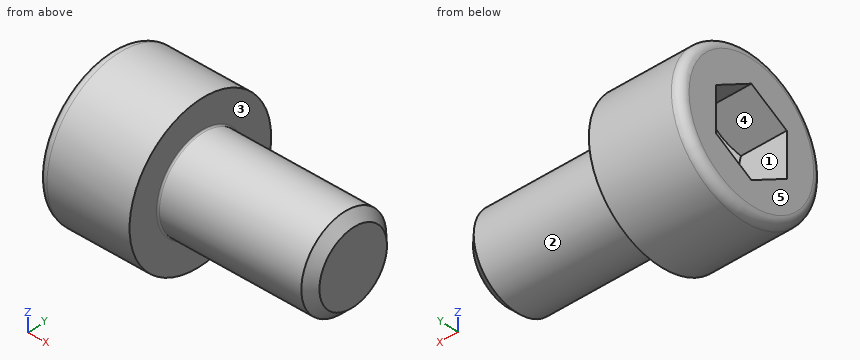
Autodesk Inventor part; units mm, degrees
ref_plane "Work Plane1" through (29, 0, 0) normal (0, -1, 0) x (1, 0, 0)
ref_plane "YZ Plane" through (0, 0, 0) normal (1, 0, 0) x (0, 1, 0)
ref_plane "XZ Plane" through (0, 0, 0) normal (0, 1, 0) x (-1, 0, 0)
sketch "Sketch1" plane through (0, 0, 0) normal (0, 0, 1) x (1, 0, 0)
  line L0 (-1.3333, 0) -> (10, 0)
  line L1 (10, 0) -> (10, 3)
  line L2 (10, 3) -> (2.5, 3)
  line L3 (2.5, 3) -> (1.8865, 3)
  line L4 (1.8865, 3) -> (0, 3)
  line L5 (0, 3) -> (0, 5)
  line L6 (0, 5) -> (-6, 5)
  line L7 (-6, 5) -> (-6, 2.8868)
  line L8 (-6, 2.8868) -> (-3, 2.8868)
  line L9 (-3, 2.8868) -> (-1.3333, 0)
  line L10 (-9.2, 0) -> (13.2, 0)
  line L11 (0, -1) -> (0, 6)
  line L12 (2.5, 3) -> (0, 3) construction
  dimension "d1" = 7.5
  dimension "d2" = 0.6136
  dimension "d3" = 6
  dimension "d4" = 3
  dimension "d5" = 60
  dimension "d6" = 6
  dimension "d7" = 6
  dimension "d8" = 5.7735
  dimension "d9" = 10
  dimension "d26" = 10
revolve "Body" add sketch "Sketch1" angle 360 about axis through (-1.3333, 0, 0) along (1, 0, 0)
sketch "Sketch2" plane through (-6, 0, 0) normal (-1, 0, 0) x (0, 0, 1)
  circle A0 centre (0, 0) radius 2.8868
  line L0 (0, -7) -> (0, 7)
  line L1 (-7, 0) -> (7, 0)
  line L2 (2.8868, 0) -> (1.4434, -2.5)
  line L3 (1.4434, -2.5) -> (-1.4434, -2.5)
  line L4 (-1.4434, -2.5) -> (-2.8868, 0)
  line L5 (-2.8868, 0) -> (-1.4434, 2.5)
  line L6 (-1.4434, 2.5) -> (1.4434, 2.5)
  line L7 (1.4434, 2.5) -> (2.8868, 0)
extrude "Slot" add sketch "Sketch2" against normal up to next contours L7 A0 | A0 L2 | L6 L0 A0 | A0 L0 L3 | L0 L6 A0 | A0 L3 L0 | L4 A0 | A0 L5
fillet "Fillet1" radius 0.6 1 edges at (-6, -5, 0)
thread "Thread"
chamfer "Chamfer1" distance 0.6135 distance2 0.6135 1 edges at (10, -3, 0) measured on face at (10, 0.705, 0.3049)
ref_plane "Work Plane1" through (29, 0, 0) normal (0, -1, 0) x (1, 0, 0)
fillet "Fillet2" radius 0.1 1 edges at (0, -3, 0)
equation "\"d1\" = GEL"
equation "\"d3\" = KOH"
equation "\"d4\" = INTI"
equation "\"d6\" = GD"
equation "\"d7\" = BDM"
equation "\"d8\" = 1.1547 * SW"
equation "\"d9\" = KOD"
equation "\"d26\" = NLG"
equation "\"d30\" = R"
equation "\"d17\" = RR"
equation "\"d13\" = GEL"
equation "\"d15\" = -0.5 * SPD + 0.5 * GD"
equation "\"d16\" = GUL"
equation "\"GD\" = NND"
equation "\"NLG\" = 10"
equation "\"GEL\" = 7.5"
equation "\"KOD\" = 10"
equation "\"KOH\" = NND"
equation "\"INTI\" = 3"
equation "\"GAL\" = 0.61345 * PTC"
equation "\"GUL\" = 0.61345 * PTC"
equation "\"BDM\" = NND"
equation "\"SW\" = 5"
equation "\"RR\" = 0.1 * NND"
equation "\"SPD\" = NND - 1.2269 * PTC"
equation "\"R\" = 0.1"
equation "\"PHH\" = 0.2"
equation "\"GD1\" = THREADDIA - 1.2269 * PTC"
equation "\"THREADDIA\" = 6"
equation "\"FAWI\" = 45deg"
equation "\"PTC\" = 1"
equation "\"KOH1\" = 5.4"
equation "\"NND\" = 6"
equation "\"TOA\" = 30deg"
equation "\"E0\" = 1.155 * SW"
properties part number "AS 1420 - 1973 - M6 x 10" material "Steel, Mild"
The listing builds one solid part. Answer for the finished solid, in the listing's coordinates (mm). Face numbers are marked on the shaded views. A direction names the side the tool comes from. Round coordinates to 2 decimals unless told otherwise and drop trailing zeros. Order: outer loops, then holes, each group sorted by start corner. A loop starts at its lowest first (then second) coordinate and runs counter-clockwise, first axis right, second up. Notation, with made-up numbers: M 53.25,34 L 66.25,34 A32 ccw 66.25,66 Z; hole C -20.75,-26.75 d5. An arc over 180 degrees is marked long. Answer in a Markdown table with one row per item. Add a question column.
1) Consider line 1 along X through (y, z) = (2.5, -2.25); line 2 along Y through (x, z) = (-2.5, 4); line 3 along Y through (x, z) = (-4.25, -0.5). Determine where each line is inside the solid, lowest interval first. Write a range as from..to.
2) The part is cut by section B-B on x = -1. Determine the outline of the cut face in (y, z).
3) Determine the mould class of the marked faces 1, 2 and 3 for opening direction Y: pulls with the +Y half, pulls with the -Y half, needs draft (parallel to the pull), parting line crosses it, or undercut.
4) Flat-ended cylindrical pins translate along their axes: pin 1 Ø1 at (y, z) = (1, 1.5) entering from -X; pin 2 Ø1.5 at (x, y) = (-2.5, 2.5) entering from -Z; pin 3 Ø1 at (x, z) = (4.5, 1) entering from -Y. Find the tip coordinate at first contact, or state that the pin passes through.
5) Which of the six approach directions +Z, -Z, +X, -X, +Y, -Y give full straight-line access (tool end or side, diameter ignored) to the marked faces 4 and 5?
6) The part is cut by section A-A on x = -3.5. Determine the outline of the cut face in (y, z).
Findings below:
| question | item | result |
|---|---|---|
| 1 | line 1 | x = -6..0 |
| 1 | line 2 | y = -3..3 |
| 1 | line 3 | y = -4.97..-2.5, 2.5..4.97 |
| 2 | outline | C 0,0 d10 |
| 3 | face 1 | undercut |
| 3 | face 2 | parting line crosses it |
| 3 | face 3 | needs draft |
| 4 | pin 1 | stops at x = -2.66 |
| 4 | pin 2 | stops at z = -4.68 |
| 4 | pin 3 | stops at y = -2.96 |
| 5 | face 4 | -X |
| 5 | face 5 | +Z, -Z, -X, +Y, -Y |
| 6 | outline | C 0,0 d10; hole M -2.5,-1.44 L 0,-2.89 L 2.5,-1.44 L 2.5,1.44 L 0,2.89 L -2.5,1.44 Z |
